Design review of the part shown in the three views and the two pictorial views. Dimensions are in mm from the part's minimum x, y and z. A direction names the side the tool comes from. Give positions to 0.01 mm unless a question says otherwise; leave off trailing zeros. Write each loop counter-clockwise with the first axis right and the second up, starting at its lowest first coordinate (ties: lowest second). Pieces come first, ordered by that corner, then holes.
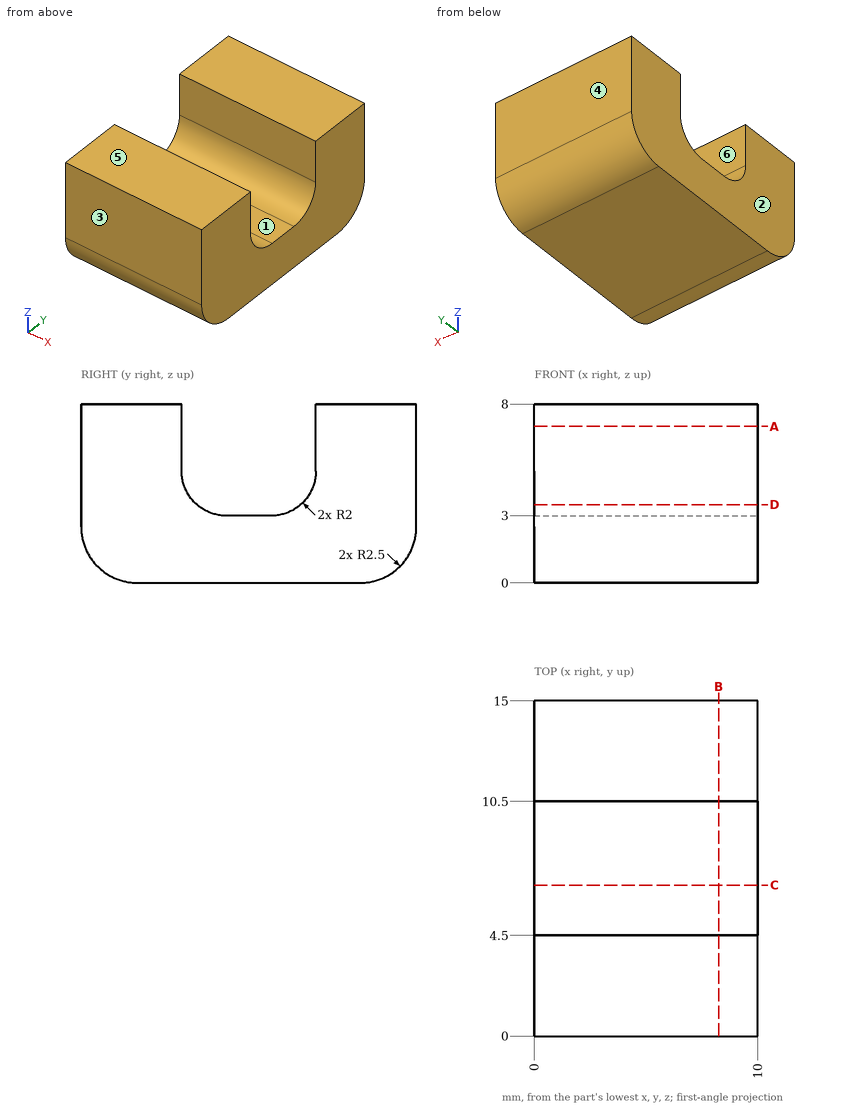
(1) Consider section B-B, the plane x = 8.25. Give the boundary of the cut face in (y, z).
Resolved:
outline: (0, 2.5) arc R2.5 ccw to (2.5, 0) - (12.5, 0) arc R2.5 ccw to (15, 2.5) - (15, 8) - (10.5, 8) - (10.5, 5) arc R2 cw to (8.5, 3) - (6.5, 3) arc R2 cw to (4.5, 5) - (4.5, 8) - (0, 8) - close
(2) Mouldability with a two-part tool opening along Y and no side actions: class the marked faces 3, 4, 5 and 6 as pulls with the +Y half, pulls with the -Y half, needs draft (parallel to the pull), parting line crosses it, or undercut.
Resolved:
face 3: pulls with the -Y half
face 4: pulls with the +Y half
face 5: needs draft
face 6: undercut
(3) To check wall thickness, follow L1, parallel to Y at x = 1, z = 5.5; L2, parallel to Z at x = 3.25, y = 7; L3, parallel to Y at x = 8.5, z = 4.5. State the ranges of each line that lie inside material, in increasing order.
Resolved:
L1: y = 0 to 4.5, 10.5 to 15
L2: z = 0 to 3
L3: y = 0 to 4.56, 10.44 to 15
(4) Consider section D-D, the plane z = 3.5. Give the boundary of the cut face in (x, y), then the cut area to 3 significant figures.
Resolved:
outline: (0, 0) - (10, 0) - (10, 5.18) - (0, 5.18) - close; (0, 9.82) - (10, 9.82) - (10, 15) - (0, 15) - close
area: 104 mm2
(5) Consider section C-C, the plane y = 6.75. Give the boundary of the cut face in (x, z), then the cut area to 3 significant figures.
Resolved:
outline: (0, 0) - (10, 0) - (10, 3) - (0, 3) - close
area: 30.0 mm2
(6) Consider section A-A, the plane z = 7. Give the boundary of the cut face in (x, y), then the cut area to 3 significant figures.
Resolved:
outline: (0, 0) - (10, 0) - (10, 4.5) - (0, 4.5) - close; (0, 10.5) - (10, 10.5) - (10, 15) - (0, 15) - close
area: 90.0 mm2
(7) Tool access review of the marked faces 1 and 2: name each direction out of +Z, -Z, +X, -X, +Y, -Y from which nothing blocks a thin tool from reaching the whole face with its end or side.
Resolved:
face 1: +Z, +X, -X
face 2: +Z, -Z, -X, +Y, -Y
(8) Clearance check with a flat-ended pin moving along its axis: P1, Ø1, axis at x = 3.5, y = 8, coming from the +Z side. State where the tip first meets the part, or that it passes through.
Resolved:
P1: stops at z = 3
